from build123d import *

# Parameters (mm, degrees)
F0_W     = 22.733
F0_H     = 5.08
F0_H_2   = 2.286
F0_W_2   = 4.9149
F0_H_3   = 15.494
F1_DEPTH = 12.192
F2_R     = 2.3495
F3_DEPTH = 2.54


with BuildPart() as f1:
    # F0 (on Top) → F1 (new body)
    with BuildSketch(Plane.XY):
        with Locations((0, 8.89)):
            Rectangle(F0_W, F0_H)
        with Locations((0, 5.207)):
            Rectangle(F0_W, F0_H_2)
        with Locations((-13.82395, 5.207)):
            Rectangle(F0_W_2, F0_H_2)
        with Locations((0, -3.683)):
            Rectangle(F0_W, F0_H_3)
        with Locations((13.82395, 5.207)):
            Rectangle(F0_W_2, F0_H_2)
    extrude(amount=F1_DEPTH)

    # F2 (on face) → F3 (join)
    with BuildSketch(Plane(origin=(0, 11.43, 0), x_dir=(-1, 0, 0), z_dir=(0, 1, 0))):
        with Locations((-6.7945, 6.096)):
            Circle(F2_R)
    extrude(amount=F3_DEPTH)


solid = f1.part
Source: CAD feature listing. Evaluate the final solid. Frame: model axes, mm. A direction names the side the tool comes from. Give positions to 0.01 mm unless a question says otherwise; leave off trailing zeros. Write each loop counter-clockwise with the first axis right and the second up, starting at its lowest first coordinate (ties: lowest second). Pieces come first, ordered by that corner, then holes. Notation, with made-up numbers: M 77.5,72.25 L 95.5,72.25 A24 ccw 95.5,104.25 Z; hole C 56.25,-17.5 d1. An arc over 180 degrees is marked long. Answer as a JSON object with one key per item and string values.
Q1. Cut plane D-D, the plane x = -13. Return the cut outline in (y, z), then the cut area to 3 significant figures.
Geometry check:
{"outline": "M 4.06,0 L 6.35,0 L 6.35,12.19 L 4.06,12.19 Z", "area": "27.9 mm^2"}
Q2. Cut plane B-B, the plane x = 7. Return the cut outline in (y, z).
Geometry check:
{"outline": "M -11.43,0 L 11.43,0 L 11.43,3.76 L 13.97,3.76 L 13.97,8.44 L 11.43,8.44 L 11.43,12.19 L -11.43,12.19 Z"}
Q3. Contact query for flat-ended pins moving along their axis: P1, Ø3.5, axis at x = -3, z = 7, coming from the +Y side; P2, Ø1.5, axis at y = 10, z = 5, coming from the -X side; P3, Ø4, axis at x = -14, z = 7.5, coming from the -Y side. Output: stop coordinate, or through.
Geometry check:
{"P1": "stops at y = 11.43", "P2": "stops at x = -11.37", "P3": "stops at y = 4.06"}
Q4. Cut plane A-A, the plane z = 2.25. Return the cut outline in (x, y), then the cut area to 3 significant figures.
Geometry check:
{"outline": "M -16.28,4.06 L -11.37,4.06 L -11.37,-11.43 L 11.37,-11.43 L 11.37,4.06 L 16.28,4.06 L 16.28,6.35 L 11.37,6.35 L 11.37,11.43 L -11.37,11.43 L -11.37,6.35 L -16.28,6.35 Z", "area": "542 mm^2"}
Q5. Access query for faces 1 (the face through (-11.366, -4, 6)), 2 (the face through (14, 4.064, 6)), 3 (the face through (-14, 6.35, 6)). Directions: +Z, -Z, +X, -X, +Y, -Y. A direction counts if a zero-diameter tool reaches every point of the face in a straight line with its end or side. Return the directions, or none.
Geometry check:
{"face 1": "+Z, -Z, -X, -Y", "face 2": "+Z, -Z, +X, -Y", "face 3": "+Z, -Z, -X, +Y"}
Q6. Cut plane C-C, the plane y = -4.75. Return the cut outline in (x, z), then the cut area to 3 significant figures.
Geometry check:
{"outline": "M -11.37,0 L 11.37,0 L 11.37,12.19 L -11.37,12.19 Z", "area": "277 mm^2"}
Q7. Ray query, line 1 along X through (y, z) = (0.5, 11); line 2 along Y through (x, z) = (8, 2.75); line 3 along Y through (x, z) = (-13.5, 5.5). Return the intervals inside material, ascending.
Geometry check:
{"line 1": "x = -11.37 to 11.37", "line 2": "y = -11.43 to 11.43", "line 3": "y = 4.06 to 6.35"}
